For this review, take the finished solid that the model builds, in its own axes (mm). Face numbers are marked on the shaded views. A direction names the side the tool comes from. Coordinates: 2 decimals unless noted, no trailing zeros. Write each loop counter-clockwise with the first axis right and the second up, starting at its lowest first coordinate (ties: lowest second). Pieces come first, ordered by that corner, then holes.
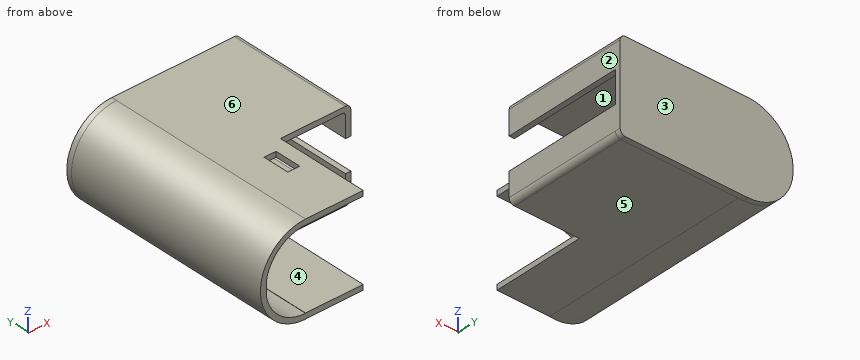
Autodesk Inventor part; units mm, degrees
ref_plane "Work Plane1" through (0, 82, 0) normal (0, 1, 0) x (1, 0, 0)
ref_plane "YZ Plane" through (0, 0, 0) normal (1, 0, 0) x (0, 1, 0)
ref_plane "XZ Plane" through (0, 0, 0) normal (0, 1, 0) x (-1, 0, 0)
sketch "Sketch1" plane through (0, 0, 0) normal (0, 1, 0) x (-1, 0, 0)
  line L0 (-15.6488, -14.9) -> (-4.1777, -14.9)
  line L1 (-4.1777, 15) -> (-13.2013, 15)
  line L2 (14.7902, 2.5) -> (14.8, 2.5)
  line L3 (14.8, 2.5) -> (14.8, -2.5)
  line L4 (14.8, -2.5) -> (14.7902, -2.5)
  arc A0 (0, -15) -> (14.7902, -2.5) centre (0, 0) ccw
  arc A1 (14.7902, 2.5) -> (0, 15) centre (0, 0) ccw
  line L5 (0.0236, 15) -> (0.0236, 15.0064)
  line L6 (0.0236, 15) -> (-4.1777, 15)
  line L7 (-4.1777, 15) -> (-4.1777, 15)
  line L8 (-0.1777, -14.9) -> (-4.1777, -14.9)
  line L9 (-4.1777, -14.9) -> (0, -14.9)
  line L10 (-4.1777, -14.9) -> (-4.1777, -14.9)
  line L11 (-13.2013, 15) -> (-46.2013, 15)
  line L12 (-15.6488, -14.9) -> (-46.2013, -14.9)
  line L13 (-46.2013, -14.9) -> (-46.2013, 15)
  arc A2 (-1.8412, -16.9) -> (0, 17) centre (0, 0) ccw
  line L14 (0, 17) -> (-48.2013, 17)
  line L15 (-48.2013, 17) -> (-48.2013, -16.9)
  line L16 (-48.2013, -16.9) -> (-1.8412, -16.9)
  line L17 (0.0236, 15) -> (0.0236, 15)
  line L18 (0, -14.9) -> (0, -15)
  point P0 (-13.2013, 0)
  point P1 (12.5, 0)
  point P2 (11.0065, 21.7068)
  point P3 (11.0065, 50.7004)
  dimension "d7" = 33
  dimension "d8" = 2
  dimension "d9" = 2
  dimension "d10" = 2
  dimension "d11" = 2
  dimension "d39" = 15
  dimension "d90" = 33.9
  dimension "d91" = 29.9
  dimension "d92" = 2
  dimension "d93" = 2
  dimension "d94" = 2.2
  dimension "d95" = 14.8
extrude "Extrusion1" add sketch "Sketch1" along normal blind 80
ref_plane "Work Plane1" through (0, 82, 0) normal (0, 1, 0) x (1, 0, 0)
sketch "Sketch3" plane through (0, 82, 0) normal (0, 1, 0) x (1, 0, 0)
  arc A0 (0, 17) -> (0, -17) centre (0, 0) ccw
  line L0 (0, -17) -> (48.2013, -17)
  line L1 (48.2013, -17) -> (48.2013, 17)
  line L2 (48.2013, 17) -> (0, 17)
  point P0 (13.2013, 0)
  point P1 (-14.9845, -166.3883)
  point P2 (-14.9845, -137.3947)
  point P3 (-26.1687, -202.0885)
extrude "Extrusion2" add sketch "Sketch3" against normal up to surface (2 mm away)
sketch "Sketch4" plane through (48.2013, 0, -16.9) normal (0, 0, -1) x (-1, 0, 0)
  point P0 (48.2013, 0)
fillet "Fillet1" radius 2 2 edges at (48.2013, 40, -16.9) (48.2013, 41, 17)
fillet "Fillet2" radius 1 2 edges at (46.2013, 40, 15) (46.2013, 40, -14.9)
fillet "Fillet3" radius 2 1 edges at (48.2013, 81, -17)
sketch "Sketch10" plane through (0, 0, 0) normal (0, -1, 0) x (1, 0, 0)
  line L0 (0, -17) -> (46.2013, -17)
  line L1 (23.9488, -17) -> (41.9488, -17)
  line L2 (41.9488, -17) -> (41.9488, -3)
  line L3 (41.9488, -3) -> (23.9488, -3)
  line L4 (23.9488, -3) -> (23.9488, -17)
  point P0 (0, 0)
  dimension "d79" = 14
  dimension "d80" = 18
sketch "Sketch11" plane through (0, 0, 0) normal (0, -1, 0) x (1, 0, 0)
  line L0 (0, 17) -> (46.2013, 17)
  line L1 (21.7013, 17) -> (48.2013, 17)
  line L2 (48.2013, 17) -> (48.2013, -16.9)
  line L3 (48.2013, -16.9) -> (21.7013, -16.9)
  line L4 (21.7013, -16.9) -> (21.7013, 17)
  line L5 (48.2013, 15) -> (48.2013, -14.9)
  point P0 (0, 0)
  dimension "d86" = 26.5
  dimension "d87" = 0
extrude "Extrusion8" cut sketch "Sketch11" against normal blind 35
sketch "Sketch12" plane through (48.2013, 82, 15) normal (1, 0, 0) x (0, 0, -1)
  line L0 (0, -47) -> (29.9, -47)
  line L1 (9, -47) -> (20.9, -47)
  line L2 (20.9, -47) -> (20.9, -2)
  line L3 (20.9, -2) -> (9, -2)
  line L4 (9, -2) -> (9, -47)
  line L5 (29.9, -2) -> (29.9, -47)
  line L6 (0, -47) -> (0, 0)
  line L7 (0, 0) -> (30, 0)
  point P0 (15, -82)
  dimension "d97" = 9
  dimension "d98" = 9
  dimension "d99" = 2
extrude "Extrusion9" cut sketch "Sketch12" against normal up to surface (2 mm away)
sketch "Sketch13" plane through (0, 0, 17) normal (0, 0, 1) x (1, 0, 0)
  line L0 (16.5, 31) -> (12, 31)
  line L1 (12, 31) -> (12, 21)
  line L2 (12, 21) -> (16.5, 21)
  line L3 (16.5, 21) -> (16.5, 31)
  line L4 (0, 0) -> (21.7013, 0)
  line L5 (0, 0) -> (0, 82)
  line L6 (0, 82) -> (46.2013, 82)
  dimension "d103" = 12
  dimension "d107" = 61
  dimension "d108" = 4.5
  dimension "d109" = 10
extrude "Extrusion10" cut sketch "Sketch13" against normal up to surface (2 mm away)
properties part number "schranka"
1) Consider section B-B (z = 0). Give the boundary of the cut face in (x, y).
2) The part is to be moulded in two halves that separate along X. For the marked faces 1, 2, 3 and 4, say which applies: pulls with the +X half, pulls with the -X half, needs draft (parallel to the pull), parting line crosses it, or undercut.
3) Tool access review of the marked faces 5 and 6: name each direction out of +Z, -Z, +X, -X, +Y, -Y from which nothing blocks a thin tool from reaching the whole face with its end or side.
4) Clearance check with flat-ended pins moving along their axes: P1, Ø4, axis at y = 51, z = 4.5, coming from the -X side; P2, Ø5.5, axis at x = 40, z = -14, coming from the -Y side; P3, Ø8, axis at y = 63.5, z = 13, coming from the -X side. State where each tip first meets the part, or that it passes through.
5) Consider section D-D (x = -5). Give the boundary of the cut face in (y, z).
6) For L1, parallel to Z at x = 44, y = 37.5; L2, parallel to Y at x = -4.5, z = -10.5; L3, parallel to X at y = 53.5, z = 13.5, list the stretches that pass through material, from the lowest coordinate up.
Results:
1. outline: (-17, 0) - (-14.8, 0) - (-14.8, 80) - (48.2, 80) - (48.2, 82) - (-17, 82) - close
2. face 1: undercut
2. face 2: pulls with the +X half
2. face 3: needs draft
2. face 4: undercut
3. face 5: -Z, +X, -Y
3. face 6: +Z, +X, -X, +Y, -Y
4. P1: stops at x = -16.82
4. P2: stops at y = 35
4. P3: stops at x = -14.42
5. outline: (0, -16.25) - (82, -16.25) - (82, 16.25) - (0, 16.25) - (0, 14.14) - (80, 14.14) - (80, -14.14) - (0, -14.14) - close
6. L1: z = -16.9 to -14.9, 15 to 17
6. L2: y = 80 to 82
6. L3: x = -10.33 to -6.54, 46.2 to 48.2
